Can you work these out from the drawing? Everything is in mm from the part's minimum corner. Round coordinates to 2 decimals unless told otherwise and drop trailing zeros. Write each loop counter-clockwise with the first axis right and the second up, starting at its lowest first coordinate (ties: lowest second). Pieces come first, ordered by that corner, then holes. Notation, with made-up numbers: (0, -7) -> (44, -7) arc R9 cw to (44, 2) -> close; hole circle Ø3 at (-18.5, 50.5). An arc over 180 degrees is marked (long way). Write item = value, one per line. Start each with the question number.
1) Imagine slicing it at B-B, the plane y = 18. Please give me the cut outline in (x, z), then the cut area to 3 significant figures.
2) Imagine slicing it at A-A, the plane x = 18. Please give me the cut outline in (y, z).
3) Imagine slicing it at C-C, the plane z = 71. Please give me the cut outline in (x, y), then the cut area to 3 significant figures.
4) Thinking about a two-plate mould opening in X: for the marked faces 1, 2 and 3, which applies, +X half, -X half, draft (parallel to the pull), parting line (faces both ways), or undercut?
5) If I drill on line 1 (Y direction, x = 18, z = 114); line 2 (Y direction, x = 18, z = 68.5); line 3 (Z direction, x = 18, y = 26), over which ranges is the centre line in solid material (lowest first)?
6) Imagine slicing it at D-D, the plane z = 126. Please give me the cut outline in (x, y), then the cut area to 3 significant figures.
7) I'm going to push flat-ended pins straight in: pin 1 (4 mm diameter, centred on x = 7, z = 46, fed in from +Y); pin 2 (8 mm diameter, centred on x = 18, z = 126, fed in from -Y); pin 3 (8 mm diameter, centred on y = 31, z = 109.5, fed in from -X); pin 4 (1 mm diameter, centred on x = 19.5, y = 21.5, fed in from +Z). Where does each tip first touch, or does it pass through?
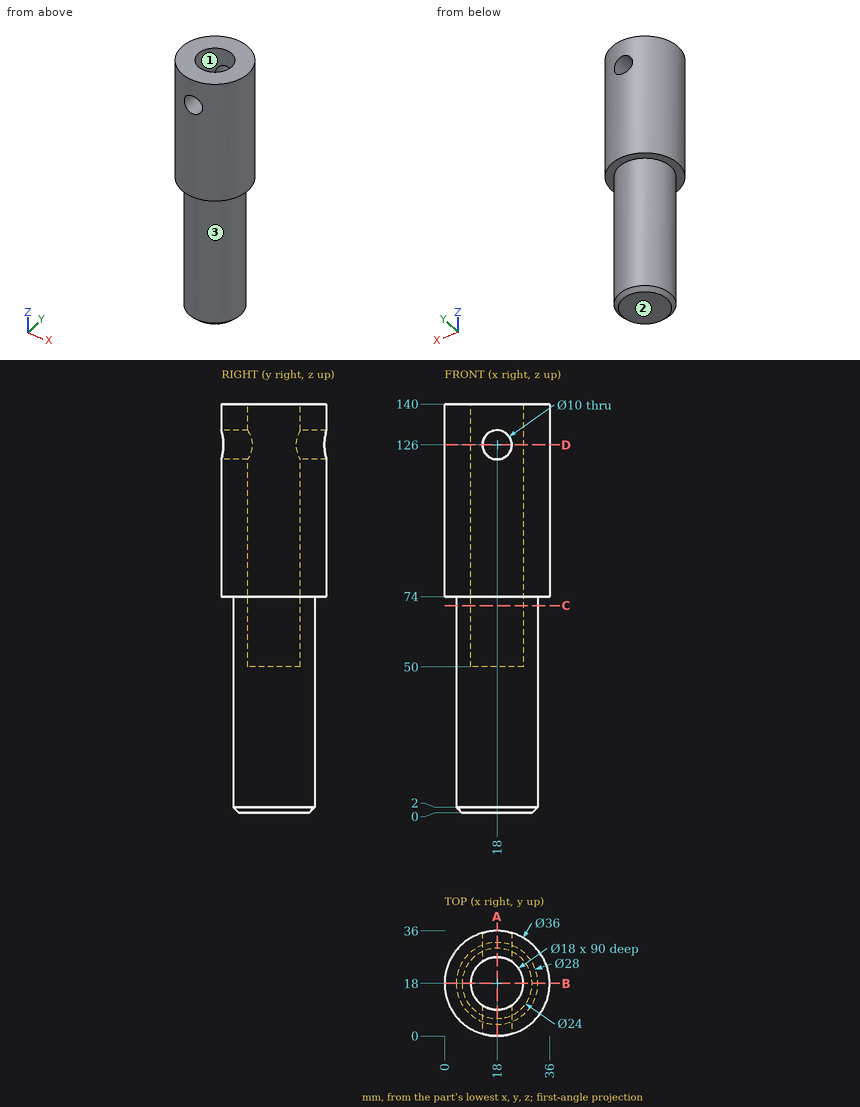
Reported:
q1.outline = (0, 74) -> (4, 74) -> (4, 2) -> (6, 0) -> (30, 0) -> (32, 2) -> (32, 74) -> (36, 74) -> (36, 140) -> (27, 140) -> (27, 50) -> (9, 50) -> (9, 140) -> (0, 140) -> close
q1.area = 2,820 mm²
q2.outline = (0, 74) -> (4, 74) -> (4, 2) -> (6, 0) -> (30, 0) -> (32, 2) -> (32, 74) -> (36, 74) -> (36, 121) -> (27, 121) -> (27, 50) -> (9, 50) -> (9, 121) -> (0, 121) -> close; (0, 131) -> (9, 131) -> (9, 140) -> (0, 140) -> close; (27, 131) -> (36, 131) -> (36, 140) -> (27, 140) -> close
q3.outline = circle Ø28 at (18, 18); hole circle Ø18 at (18, 18)
q3.area = 361 mm²
q4.face_1 = undercut
q4.face_2 = draft
q4.face_3 = parting line
q5.line_1 = 0 to 9, 27 to 36
q5.line_2 = 4 to 9, 27 to 32
q5.line_3 = 0 to 50
q6.outline = (13, 0.71) -> (13, 10.52) arc R9 cw to (13, 25.48) -> (13, 35.29) arc R18 ccw to start; (23, 0.71) arc R18 ccw to (23, 35.29) -> (23, 25.48) arc R9 cw to (23, 10.52) -> close
q6.area = 578 mm²
q7.pin_1 = 28.72
q7.pin_2 = through
q7.pin_3 = 2.41
q7.pin_4 = 50
